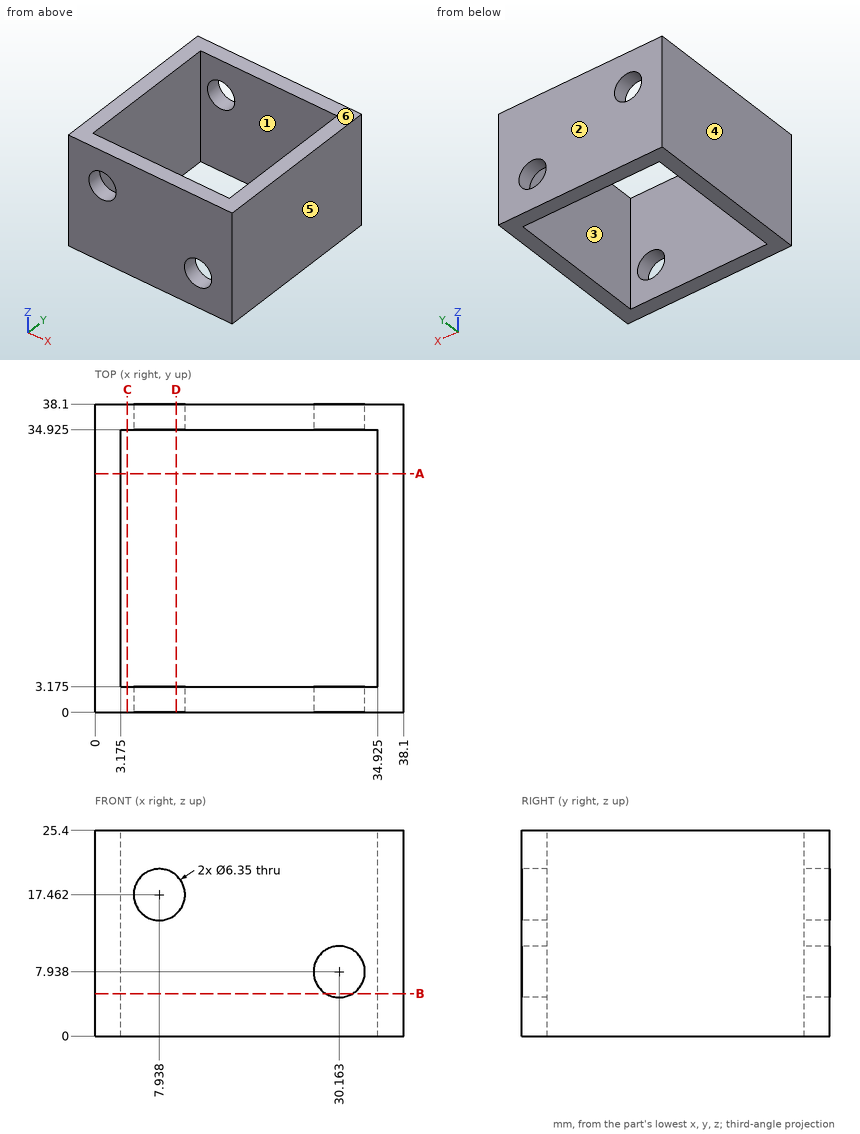
Drawing for the job (mm, zero at the part's lowest x, y, z). A direction names the side the tool comes from. Give positions to 0.01 mm unless a question says otherwise; leave off trailing zeros. Loops run counter-clockwise (first coordinate to the right, second up) from the corner with the lowest first, then second, coordinate; pieces in that order, holes last. Notation, with made-up numbers: (42, -29.75) - (94, -29.75) arc R26 cw to (94, -0.75) - close; hole circle Ø9 at (81.5, 24.5). An arc over 180 degrees is marked (long way). Write item = value, one per line. Start each with the question number.
1) Pull direction X, two halves, no side cores. Call the marked faces 3, 4, 5 and 6: +X half, -X half, draft (parallel to the pull), parting line (faces both ways), or undercut.
2) Band-saw the part on B-B on z = 5.25. Give the cut face in (x, y) (1 decimal), plus the area to 3 significant figures.
3) Drop flat-ended pins along their axis: pin 1 Ø6 at (x, y) = (6.5, 29.5) entering from +Z; pin 2 Ø10 at (x, z) = (7.94, 17.46) entering from +Y. Give the stop position or say it passes through.
4) Probe probe 1 along X at (y, z) = (30, 19) (1 decimal). List the from-to ranges inside material, lowest first. Write a range as from..to.
5) Band-saw the part on D-D on x = 10. Give the cut face in (y, z) (1 decimal), plus the area to 3 significant figures.
6) Band-saw the part on A-A on y = 29.5. Give the cut face in (x, z) (1 decimal), plus the area to 3 significant figures.
7) Tool access for the marked faces 1 and 2: list every direction of +Z, -Z, +X, -X, +Y, -Y with a clear straight run to the whole face (end or side of a thin tool).
Final values:
q1.face_3 = undercut
q1.face_4 = -X half
q1.face_5 = +X half
q1.face_6 = draft
q2.outline = (0, 0) - (28.5, 0) - (28.5, 3.2) - (3.2, 3.2) - (3.2, 34.9) - (28.5, 34.9) - (28.5, 38.1) - (0, 38.1) - close; (31.9, 0) - (38.1, 0) - (38.1, 38.1) - (31.9, 38.1) - (31.9, 34.9) - (34.9, 34.9) - (34.9, 3.2) - (31.9, 3.2) - close
q2.area = 422 mm²
q3.pin_1 = through
q3.pin_2 = 38.1
q4.probe_1 = 0..3.2, 34.9..38.1
q5.outline = (0, 0) - (3.2, 0) - (3.2, 15) - (0, 15) - close; (0, 19.9) - (3.2, 19.9) - (3.2, 25.4) - (0, 25.4) - close; (34.9, 0) - (38.1, 0) - (38.1, 15) - (34.9, 15) - close; (34.9, 19.9) - (38.1, 19.9) - (38.1, 25.4) - (34.9, 25.4) - close
q5.area = 131 mm²
q6.outline = (0, 0) - (3.2, 0) - (3.2, 25.4) - (0, 25.4) - close; (34.9, 0) - (38.1, 0) - (38.1, 25.4) - (34.9, 25.4) - close
q6.area = 161 mm²
q7.face_1 = +Z, -Z
q7.face_2 = +Z, -Z, +X, -X, +Y
